from build123d import *
from OCP.BRepFilletAPI import BRepFilletAPI_MakeChamfer

# Parameters (mm, degrees)
SKETCH1_W           = 50.8
SKETCH1_H           = 25.4
BOSS_EXTRUDE1_DEPTH = 12.7
HOLE1_D             = 4.9276
CHAMFER1_SIZE       = 1.9685
CHAMFER1_SIZE2      = 2.264500221


with BuildPart() as part:
    # Sketch1 → Boss-Extrude1 (new body)
    with BuildSketch(Plane(origin=(0, 6.35, 0), x_dir=(1, 0, 0), z_dir=(0, 1, 0))):
        Rectangle(SKETCH1_W, SKETCH1_H)
    extrude(amount=-BOSS_EXTRUDE1_DEPTH)

    # Hole1 (through all)
    with Locations(Plane(origin=(0, 6.35, 0), x_dir=(1, 0, 0), z_dir=(0, 1, 0))):
        with Locations((-12.7, 0), (12.7, 0)):
            Hole(HOLE1_D / 2)

    # Chamfer1: one chamfer whose edges measure the first distance from different faces: ONE call of the kernel's chamfer builder (chamfer() names one face for all edges)
    chamfer1_edges_1 = [part.edges().sort_by_distance(p)[0] for p in [
        (15.1638, 6.35, 0),
        (-10.2362, 6.35, 0),
    ]]
    chamfer1_side_1 = [part.faces().sort_by_distance(p)[0] for p in [
        (0, 6.35, 0),
    ]]
    chamfer1_edges_2 = [part.edges().sort_by_distance(p)[0] for p in [
        (15.1638, -6.35, 0),
    ]]
    chamfer1_side_2 = [part.faces().sort_by_distance(p)[0] for p in [
        (15.1638, 0, 0),
    ]]
    chamfer1_edges_3 = [part.edges().sort_by_distance(p)[0] for p in [
        (-10.2362, -6.35, 0),
    ]]
    chamfer1_side_3 = [part.faces().sort_by_distance(p)[0] for p in [
        (-10.2362, 0, 0),
    ]]
    chamfer1 = BRepFilletAPI_MakeChamfer(part.part.solid().wrapped)
    for e in chamfer1_edges_1:
        chamfer1.Add(CHAMFER1_SIZE, CHAMFER1_SIZE2, e.wrapped, chamfer1_side_1[0].wrapped)  # the first distance lies on this face
    for e in chamfer1_edges_2:
        chamfer1.Add(CHAMFER1_SIZE, CHAMFER1_SIZE2, e.wrapped, chamfer1_side_2[0].wrapped)  # the first distance lies on this face
    for e in chamfer1_edges_3:
        chamfer1.Add(CHAMFER1_SIZE, CHAMFER1_SIZE2, e.wrapped, chamfer1_side_3[0].wrapped)  # the first distance lies on this face
    add(Compound.cast(chamfer1.Shape()), mode=Mode.REPLACE)


solid = part.part
The listing builds one solid part. Answer for the finished solid, in the listing's coordinates (mm). Coordinates: 2 decimals unless noted, no trailing zeros. Order: outer loops, then holes, each group sorted by start corner. A loop starts at its lowest first (then second) coordinate and runs counter-clockwise, first axis right, second up. Notation, with made-up numbers: M 17,-6.75 L 35,-6.75 A6 ccw 35,3.25 Z; hole C 8,11 d1. An arc over 180 degrees is marked long. Use CSV: the item, a comma, the result in double quotes.
Q1. Section B-B (x = 12.7) is taken. Determine the outline of the cut face in (y, z).
Here are the results:
outline,"M -6.35,-12.7 L 6.35,-12.7 L 6.35,-4.43 L 4.09,-2.46 L -4.38,-2.46 L -6.35,-4.73 Z; M -6.35,4.73 L -4.38,2.46 L 4.09,2.46 L 6.35,4.43 L 6.35,12.7 L -6.35,12.7 Z"
Q2. Section A-A (z = 0) is taken. Determine the outline of the cut face in (x, y), then the cut area to 3 significant figures.
Here are the results:
outline,"M -25.4,-6.35 L -17.43,-6.35 L -15.16,-4.38 L -15.16,4.09 L -17.13,6.35 L -25.4,6.35 Z; M -10.24,-4.38 L -7.97,-6.35 L 7.97,-6.35 L 10.24,-4.38 L 10.24,4.09 L 8.27,6.35 L -8.27,6.35 L -10.24,4.09 Z; M 15.16,-4.38 L 17.43,-6.35 L 25.4,-6.35 L 25.4,6.35 L 17.13,6.35 L 15.16,4.09 Z"
area,"502 mm2"
Q3. Straight lines are drawn through the part: L1, parallel to X at y = -1.25, z = 0; L2, parallel to Z at x = 12.7, y = 1.5; L3, parallel to Z at x = 14, y = 5. For each, find the intervals that lie inside material, in ascending order.
Here are the results:
L1,"-25.4 to -15.16, -10.24 to 10.24, 15.16 to 25.4"
L2,"-12.7 to -2.46, 2.46 to 12.7"
L3,"-12.7 to -2.99, 2.99 to 12.7"
Q4. Determine the mould class of faces 1 (the flat face through (-25.4, 0, 0)), 2 (the conical face through (14.62, -4.505, -1.761)), 3 (the flat face through (0, 0, -12.7)) for opening direction X: pulls with the +X half, pulls with the -X half, needs draft (parallel to the pull), parting line crosses it, or undercut.
Here are the results:
face 1,"pulls with the -X half"
face 2,"undercut"
face 3,"needs draft"
Q5. Section C-C (y = -2.5) is taken. Determine the outline of the cut face in (x, z).
Here are the results:
outline,"M -25.4,-12.7 L 25.4,-12.7 L 25.4,12.7 L -25.4,12.7 Z; hole C -12.7,0 d4.93; hole C 12.7,0 d4.93"
Q6. Given pin 1 Ø4.5 at (x, z) = (-12.7, 0) entering from +Y; pin 2 Ø6.5 at (x, z) = (12.7, 0) entering from -Y, each flat-ended and moving along its own axis, determine where each tip first touches the part or whether it passes through.
Here are the results:
pin 1,"through"
pin 2,"y = -5.06"
